Build history of the part. All positions in model axes, mm. Face numbers are marked on the shaded views. A direction names the side the tool comes from. Coordinates: 2 decimals unless noted, no trailing zeros. Order: outer loops, then holes, each group sorted by start corner. A loop starts at its lowest first (then second) coordinate and runs counter-clockwise, first axis right, second up. Notation, with made-up numbers: M 30,-30.75 L 57,-30.75 A15 ccw 57,-20.75 Z; hole C 21.5,72 d3. An arc over 180 degrees is marked long. Write item = value, one per line. Start each with the question number.
Q1. Band-saw the part on C-C on z = -4. Write the cut outline in (x, y).
Q2. Drill centre lines: probe 1 along Y at (x, z) = (-22.5, 23.6); probe 2 along Y at (x, z) = (-22.5, -26.7); probe 3 along Z at (x, y) = (-36, 11). Where is each one in solid material? Low to high.
Q3. Band-saw the part on B-B on z = -37.5. Write the cut outline in (x, y).
Q4. Band-saw the part on D-D on z = 19.5. Write the cut outline in (x, y), plus the area to 3 significant figures.
Q5. Pin check, flat tips, straight feed: P1, Ø7, axis at x = -20.5, z = 8.5, coming from the +Y side; P2, Ø1, axis at x = 1.5, y = 23.5, coming from the -Z side; P3, Ø6, axis at y = 28.5, z = -16.5, coming from the -X side; P4, Ø5, axis at y = 25.5, z = -10, coming from the -X side. Stop position of each tip, or through.
Q6. Pull direction Z, two halves, no side cores. Call the marked faces 4, 5, 6 and 7: released by +Z, released by -Z, zero draft, split by the parting line, or undercut.
Q7. 3-axis set-ups, long thin cutter, end or side, ignore diameter. For the marked faces 1, 2 and 3: which of +Z, -Z, +X, -X, +Y, -Y reach the whole face in a straight line?
Q8. Band-saw the part on A-A on y = 8. Write the cut outline in (x, z).
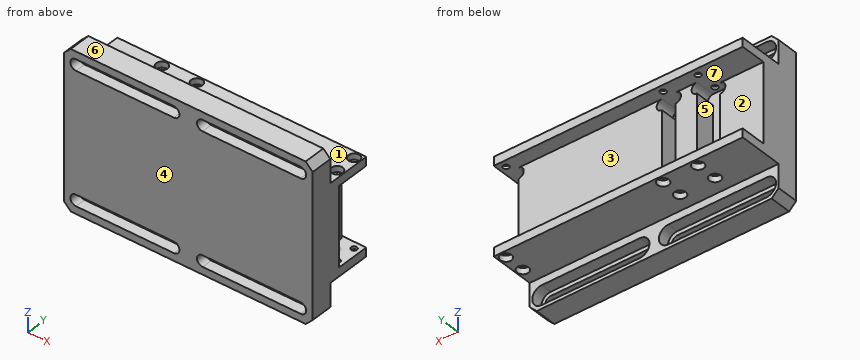
```python
from build123d import *

# Parameters (mm, degrees)
SKETCH1_W                                      = 142.5
SKETCH1_H                                      = 90
BOSS_EXTRUDE1_DEPTH                            = 12.5
CHAMFER1_SIZE                                  = 4
SKETCH3_W                                      = 142.5
SKETCH3_H                                      = 55.2
BOSS_EXTRUDE2_DEPTH                            = 25.5
SKETCH7_W                                      = 142.5
SKETCH7_H                                      = 45.2
CUT_EXTRUDE4_DEPTH                             = 8
SKETCH8_W                                      = 7.7
SKETCH8_H                                      = 32.8
SKETCH8_H_2                                    = 6.2
SKETCH8_H_3                                    = 45.2
CUT_EXTRUDE5_DEPTH                             = 11.5
SKETCH9_W                                      = 24.9
SKETCH9_H                                      = 45.2
CUT_EXTRUDE6_DEPTH                             = 6.75
CBORE_START                                    = 24.2
CBORE_FOR_M3_HEX_SOCKET_HEAD_CAP_SCR_2_R       = 3.25
CBORE_FOR_M3_HEX_SOCKET_HEAD_CAP_SCREW1_DEPTH  = 3.4
CBORE_START_2                                  = 22.6
CBORE_FOR_M3_HEX_SOCKET_HEAD_CAP_SCR_3_O_R     = 1.7
CBORE_FOR_M3_HEX_SOCKET_HEAD_CAP_SCR_3_DEPTH   = 1.6
CBORE_SLOT_FOR_M6_HEX_SOCKET_HEAD_CAP_SC_DEPTH = 12.5
CBORE_START_3                                  = 6.1
CBORE_SLOT_FOR_M6_HEX_SOCKET_HEAD_CA_3_DEPTH   = 6.4


# Read off the part's stored shape, not the designer's step: CBORE for M3 Hex Socket Head Cap Screw1, CBORE SLOT for M6 Hex Socket Head Cap Screw1
with BuildPart() as part:
    # Sketch1 → Boss-Extrude1 (new body)
    with BuildSketch(Plane(origin=(0, 0, 0), x_dir=(1, 0, 0), z_dir=(0, 1, 0))):
        Rectangle(SKETCH1_W, SKETCH1_H)
    extrude(amount=BOSS_EXTRUDE1_DEPTH)

    # Chamfer1
    chamfer1_edges = [part.edges().sort_by_distance(p)[0] for p in [
        (-71.25, 6.25, 45),
        (-71.25, 6.25, -45),
        (71.25, 6.25, -45),
        (71.25, 6.25, 45),
    ]]
    chamfer(chamfer1_edges, length=CHAMFER1_SIZE)

    # Sketch3 → Boss-Extrude2 (add)
    with BuildSketch(Plane(origin=(0, 12.5, 0), x_dir=(1, 0, 0), z_dir=(0, 1, 0))):
        Rectangle(SKETCH3_W, SKETCH3_H)
    extrude(amount=BOSS_EXTRUDE2_DEPTH)

    # Sketch7 → Cut-Extrude4 (cut)
    with BuildSketch(Plane(origin=(0, 38, 0), x_dir=(1, 0, 0), z_dir=(0, 1, 0))):
        Rectangle(SKETCH7_W, SKETCH7_H)
    extrude(amount=-CUT_EXTRUDE4_DEPTH, mode=Mode.SUBTRACT)

    # Sketch8 → Cut-Extrude5 (cut)
    with BuildSketch(Plane(origin=(0, 30, 0), x_dir=(1, 0, 0), z_dir=(0, 1, 0))):
        with BuildLine():
            ThreePointArc((-46.35, 22.6), (-49.45, 19.5), (-46.35, 16.4))
            Line((-46.35, 16.4), (-46.35, 22.6))
        make_face()
        with BuildLine():
            Line((-38.65, 22.6), (-38.65, 16.4))
            ThreePointArc((-38.65, 16.4), (-35.55, 19.5), (-38.65, 22.6))
        make_face()
        with Locations((-42.5, 0)):
            Rectangle(SKETCH8_W, SKETCH8_H)
        with Locations((-42.5, 19.5)):
            Rectangle(SKETCH8_W, SKETCH8_H_2)
        with BuildLine():
            ThreePointArc((-46.35, -16.4), (-49.45, -19.5), (-46.35, -22.6))
            Line((-46.35, -22.6), (-46.35, -16.4))
        make_face()
        with BuildLine():
            Line((-38.65, -16.4), (-38.65, -22.6))
            ThreePointArc((-38.65, -22.6), (-35.55, -19.5), (-38.65, -16.4))
        make_face()
        with Locations((-42.5, -19.5)):
            Rectangle(SKETCH8_W, SKETCH8_H_2)
        with Locations((-22.5, 0)):
            Rectangle(SKETCH8_W, SKETCH8_H_3)
        with BuildLine():
            Line((-26.35, 16.4), (-18.65, 16.4))
            ThreePointArc((-18.65, 16.4), (-15.55, 19.5), (-18.65, 22.6))
            Line((-18.65, 22.6), (-26.35, 22.6))
            ThreePointArc((-26.35, 22.6), (-29.45, 19.5), (-26.35, 16.4))
        make_face()
        with BuildLine():
            Line((-26.35, -22.6), (-18.65, -22.6))
            ThreePointArc((-18.65, -22.6), (-15.55, -19.5), (-18.65, -16.4))
            Line((-18.65, -16.4), (-26.35, -16.4))
            ThreePointArc((-26.35, -16.4), (-29.45, -19.5), (-26.35, -22.6))
        make_face()
        with Locations((67.5, 0)):
            Rectangle(SKETCH8_W, SKETCH8_H_3)
        with BuildLine():
            Line((63.65, 16.4), (71.35, 16.4))
            ThreePointArc((71.35, 16.4), (74.45, 19.5), (71.35, 22.6))
            Line((71.35, 22.6), (63.65, 22.6))
            ThreePointArc((63.65, 22.6), (60.55, 19.5), (63.65, 16.4))
        make_face()
        with BuildLine():
            Line((63.65, -22.6), (71.35, -22.6))
            ThreePointArc((71.35, -22.6), (74.45, -19.5), (71.35, -16.4))
            Line((71.35, -16.4), (63.65, -16.4))
            ThreePointArc((63.65, -16.4), (60.55, -19.5), (63.65, -22.6))
        make_face()
    extrude(amount=-CUT_EXTRUDE5_DEPTH, mode=Mode.SUBTRACT)

    # Sketch9 → Cut-Extrude6 (cut)
    with BuildSketch(Plane(origin=(0, 30, 0), x_dir=(1, 0, 0), z_dir=(0, 1, 0))):
        with Locations((-58.8, 0)):
            Rectangle(SKETCH9_W, SKETCH9_H)
    extrude(amount=-CUT_EXTRUDE6_DEPTH, mode=Mode.SUBTRACT)

    # CBORE for M3 Hex Socket Head Cap Scr 2 → CBORE for M3 Hex Socket Head Cap Screw1 (cut)
    with BuildSketch(Plane.XY.offset(CBORE_START)):
        with Locations((-42.5, 34)):
            Circle(CBORE_FOR_M3_HEX_SOCKET_HEAD_CAP_SCR_2_R)
        with Locations((-42.5, 22)):
            Circle(CBORE_FOR_M3_HEX_SOCKET_HEAD_CAP_SCR_2_R)
        with Locations((-22.5, 22)):
            Circle(CBORE_FOR_M3_HEX_SOCKET_HEAD_CAP_SCR_2_R)
        with Locations((-22.5, 34)):
            Circle(CBORE_FOR_M3_HEX_SOCKET_HEAD_CAP_SCR_2_R)
        with Locations((67.5, 22)):
            Circle(CBORE_FOR_M3_HEX_SOCKET_HEAD_CAP_SCR_2_R)
        with Locations((67.5, 34)):
            Circle(CBORE_FOR_M3_HEX_SOCKET_HEAD_CAP_SCR_2_R)
    cbore_for_m3_hex_socket_head_cap_screw1 = extrude(amount=CBORE_FOR_M3_HEX_SOCKET_HEAD_CAP_SCREW1_DEPTH, mode=Mode.SUBTRACT)

    # CBORE for M3 Hex Socket Head Cap Scr 3 o → CBORE for M3 Hex Socket Head Cap Scr 3 (cut)
    with BuildSketch(Plane.XY.offset(CBORE_START_2)):
        with Locations((-42.5, 34)):
            Circle(CBORE_FOR_M3_HEX_SOCKET_HEAD_CAP_SCR_3_O_R)
        with Locations((-42.5, 22)):
            Circle(CBORE_FOR_M3_HEX_SOCKET_HEAD_CAP_SCR_3_O_R)
        with Locations((-22.5, 22)):
            Circle(CBORE_FOR_M3_HEX_SOCKET_HEAD_CAP_SCR_3_O_R)
        with Locations((-22.5, 34)):
            Circle(CBORE_FOR_M3_HEX_SOCKET_HEAD_CAP_SCR_3_O_R)
        with Locations((67.5, 22)):
            Circle(CBORE_FOR_M3_HEX_SOCKET_HEAD_CAP_SCR_3_O_R)
        with Locations((67.5, 34)):
            Circle(CBORE_FOR_M3_HEX_SOCKET_HEAD_CAP_SCR_3_O_R)
    cbore_for_m3_hex_socket_head_cap_scr_3 = extrude(amount=CBORE_FOR_M3_HEX_SOCKET_HEAD_CAP_SCR_3_DEPTH, mode=Mode.SUBTRACT)

    # Mirror1: CBORE for M3 Hex Socket Head Cap Screw1, CBORE for M3 Hex Socket Head Cap Scr 3 across plane
    add(cbore_for_m3_hex_socket_head_cap_screw1.mirror(Plane.XY), mode=Mode.SUBTRACT)
    add(cbore_for_m3_hex_socket_head_cap_scr_3.mirror(Plane.XY), mode=Mode.SUBTRACT)

    # CBORE SLOT for M6 Hex Socket Head Ca 2 → CBORE SLOT for M6 Hex Socket Head Cap Screw1 (cut)
    with BuildSketch(Plane(origin=(0, 0, 0), x_dir=(1, 0, 0), z_dir=(0, 1, 0))):
        with BuildLine():
            Line((8.2, -40.7), (64.3, -40.7))
            ThreePointArc((64.3, -40.7), (67.5, -37.5), (64.3, -34.3))
            Line((64.3, -34.3), (8.2, -34.3))
            ThreePointArc((8.2, -34.3), (5, -37.5), (8.2, -40.7))
        make_face()
        with BuildLine():
            ThreePointArc((-8.2, -40.7), (-5, -37.5), (-8.2, -34.3))
            Line((-8.2, -34.3), (-64.3, -34.3))
            ThreePointArc((-64.3, -34.3), (-67.5, -37.5), (-64.3, -40.7))
            Line((-64.3, -40.7), (-8.2, -40.7))
        make_face()
        with BuildLine():
            Line((8.2, 34.3), (64.3, 34.3))
            ThreePointArc((64.3, 34.3), (67.5, 37.5), (64.3, 40.7))
            Line((64.3, 40.7), (8.2, 40.7))
            ThreePointArc((8.2, 40.7), (5, 37.5), (8.2, 34.3))
        make_face()
        with BuildLine():
            ThreePointArc((-8.2, 34.3), (-5, 37.5), (-8.2, 40.7))
            Line((-8.2, 40.7), (-64.3, 40.7))
            ThreePointArc((-64.3, 40.7), (-67.5, 37.5), (-64.3, 34.3))
            Line((-64.3, 34.3), (-8.2, 34.3))
        make_face()
    extrude(amount=CBORE_SLOT_FOR_M6_HEX_SOCKET_HEAD_CAP_SC_DEPTH, mode=Mode.SUBTRACT)

    # CBORE SLOT for M6 Hex Socket Head Ca 3 o → CBORE SLOT for M6 Hex Socket Head Ca 3 (cut)
    # profile 1 of 4: a face of its own
    with BuildSketch(Plane(origin=(0, 0, 0), x_dir=(1, 0, 0), z_dir=(0, 1, 0)).offset(CBORE_START_3)):
        with BuildLine():
            Line((8.2, -43), (64.3, -43))
            ThreePointArc((64.3, -43), (69.8, -37.5), (64.3, -32))
            Line((64.3, -32), (8.2, -32))
            ThreePointArc((8.2, -32), (2.7, -37.5), (8.2, -43))
        make_face()
        with BuildLine():
            ThreePointArc((64.3, -34.3), (67.5, -37.5), (64.3, -40.7))
            Line((64.3, -40.7), (8.2, -40.7))
            ThreePointArc((8.2, -40.7), (5, -37.5), (8.2, -34.3))
            Line((8.2, -34.3), (64.3, -34.3))
        make_face(mode=Mode.SUBTRACT)
    # profile 2 of 4: a face of its own
    with BuildSketch(Plane(origin=(0, 0, 0), x_dir=(1, 0, 0), z_dir=(0, 1, 0)).offset(CBORE_START_3)):
        with BuildLine():
            ThreePointArc((-8.2, -43), (-2.7, -37.5), (-8.2, -32))
            Line((-8.2, -32), (-64.3, -32))
            ThreePointArc((-64.3, -32), (-69.8, -37.5), (-64.3, -43))
            Line((-64.3, -43), (-8.2, -43))
        make_face()
        with BuildLine():
            Line((-64.3, -34.3), (-8.2, -34.3))
            ThreePointArc((-8.2, -34.3), (-5, -37.5), (-8.2, -40.7))
            Line((-8.2, -40.7), (-64.3, -40.7))
            ThreePointArc((-64.3, -40.7), (-67.5, -37.5), (-64.3, -34.3))
        make_face(mode=Mode.SUBTRACT)
    # profile 3 of 4: a face of its own
    with BuildSketch(Plane(origin=(0, 0, 0), x_dir=(1, 0, 0), z_dir=(0, 1, 0)).offset(CBORE_START_3)):
        with BuildLine():
            Line((8.2, 32), (64.3, 32))
            ThreePointArc((64.3, 32), (69.8, 37.5), (64.3, 43))
            Line((64.3, 43), (8.2, 43))
            ThreePointArc((8.2, 43), (2.7, 37.5), (8.2, 32))
        make_face()
        with BuildLine():
            ThreePointArc((64.3, 40.7), (67.5, 37.5), (64.3, 34.3))
            Line((64.3, 34.3), (8.2, 34.3))
            ThreePointArc((8.2, 34.3), (5, 37.5), (8.2, 40.7))
            Line((8.2, 40.7), (64.3, 40.7))
        make_face(mode=Mode.SUBTRACT)
    # profile 4 of 4: a face of its own
    with BuildSketch(Plane(origin=(0, 0, 0), x_dir=(1, 0, 0), z_dir=(0, 1, 0)).offset(CBORE_START_3)):
        with BuildLine():
            ThreePointArc((-8.2, 32), (-2.7, 37.5), (-8.2, 43))
            Line((-8.2, 43), (-64.3, 43))
            ThreePointArc((-64.3, 43), (-69.8, 37.5), (-64.3, 32))
            Line((-64.3, 32), (-8.2, 32))
        make_face()
        with BuildLine():
            Line((-64.3, 40.7), (-8.2, 40.7))
            ThreePointArc((-8.2, 40.7), (-5, 37.5), (-8.2, 34.3))
            Line((-8.2, 34.3), (-64.3, 34.3))
            ThreePointArc((-64.3, 34.3), (-67.5, 37.5), (-64.3, 40.7))
        make_face(mode=Mode.SUBTRACT)
    extrude(amount=CBORE_SLOT_FOR_M6_HEX_SOCKET_HEAD_CA_3_DEPTH, mode=Mode.SUBTRACT)


solid = part.part
```
Recorded:
q1.outline = M -71.25,0 L 71.25,0 L 71.25,18.5 L 63.65,18.5 L 63.65,30 L -18.65,30 L -18.65,18.5 L -26.35,18.5 L -26.35,30 L -38.65,30 L -38.65,18.5 L -46.35,18.5 L -46.35,23.25 L -71.25,23.25 Z
q2.probe_1 = 0 to 20.3, 23.7 to 32.3, 35.7 to 38
q2.probe_2 = 0 to 18.75, 25.25 to 30.75, 37.25 to 38
q2.probe_3 = -45 to -43, -32 to 32, 43 to 45
q3.outline = M -71.25,0 L -67.5,0 L -67.5,6.1 L -69.8,6.1 L -69.8,12.5 L -71.25,12.5 Z; M -5,0 L 5,0 L 5,6.1 L 2.7,6.1 L 2.7,12.5 L -2.7,12.5 L -2.7,6.1 L -5,6.1 Z; M 67.5,0 L 71.25,0 L 71.25,12.5 L 69.8,12.5 L 69.8,6.1 L 67.5,6.1 Z
q4.outline = M -71.25,0 L 71.25,0 L 71.25,18.5 L 60.55,18.5 L 60.55,30 L -15.55,30 L -15.55,18.5 L -29.45,18.5 L -29.45,30 L -35.55,30 L -35.55,18.5 L -49.45,18.5 L -49.45,23.25 L -71.25,23.25 Z
q4.area = 3,690 mm2
q5.P1 = 30
q5.P2 = -27.6
q5.P3 = -38.65
q5.P4 = -71.25
q6.face_4 = zero draft
q6.face_5 = undercut
q6.face_6 = released by +Z
q6.face_7 = undercut
q7.face_1 = +Z, +X, -X, +Y
q7.face_2 = -X, +Y
q7.face_3 = +X, -X, +Y
q8.outline = M -71.25,-41 L -67.25,-45 L 67.25,-45 L 71.25,-41 L 71.25,41 L 67.25,45 L -67.25,45 L -71.25,41 Z; hole M -64.3,-43 L -8.2,-43 A5.5 ccw -8.2,-32 L -64.3,-32 A5.5 ccw Z; hole M -64.3,32 L -8.2,32 A5.5 ccw -8.2,43 L -64.3,43 A5.5 ccw Z; hole M 8.2,-43 L 64.3,-43 A5.5 ccw 64.3,-32 L 8.2,-32 A5.5 ccw Z; hole M 8.2,32 L 64.3,32 A5.5 ccw 64.3,43 L 8.2,43 A5.5 ccw Z
